Source: CAD feature listing. Evaluate the final solid. Frame: model axes, mm. A direction names the side the tool comes from. Coordinates: 2 decimals unless noted, no trailing zeros. Order: outer loops, then holes, each group sorted by start corner. A loop starts at its lowest first (then second) coordinate and runs counter-clockwise, first axis right, second up.
```python
from build123d import *

# Parameters (mm, degrees)
F1_DEPTH  = 50.8
F2_R      = 3.9624
F3_SIZE   = 6.35
F5_DEPTH  = 44.451
F7_D      = 13.0302
F9_DEPTH  = 69.851
F10_R     = 29.21
F11_DEPTH = 29.591
F12_SIZE  = 4.19099
F14_DEPTH = 14.9870001
F16_DEPTH = 16.764
F17_R     = 6.35
F18_DEPTH = 69.851


# Not quite as in the source:
# - a fillet or chamfer is up to 0.001 mm smaller than in the source, because OpenCascade refuses the exact size


with BuildPart() as f1:
    # F0 (on Top) → F1 (new body)
    with BuildSketch(Plane.XY):
        Polygon((44.45, 120.65), (0, 120.65), (0, 0), (0, -21.59), (0, -73.9648), (14.986, -73.9648), (14.986, 26.2809675187), (31.75, 26.2809675187), (31.75, -21.59), (69.85, -21.59), (69.85, 0), (44.45, 0), align=None)
    extrude(amount=F1_DEPTH)

    # F2
    f2_edges = [f1.edges().sort_by_distance(p)[0] for p in [
        (44.45, 0, 25.4),
        (14.986, 26.280968, 25.4),
        (31.75, 26.280968, 25.4),
    ]]
    fillet(f2_edges, radius=F2_R)

    # F3
    f3_edges = [f1.edges().sort_by_distance(p)[0] for p in [
        (22.225, 120.65, 50.8),
        (22.225, 120.65, 0),
    ]]
    chamfer(f3_edges, length=F3_SIZE)

    # F4 (on face) → F5 (cut, through all)
    with BuildSketch(Plane.YZ.offset(44.45)):
        with BuildLine():
            Line((120.65, 38.0365), (107.8865, 38.0365))
            ThreePointArc((107.8865, 38.0365), (95.25, 25.4), (107.8865, 12.7635))
            Line((107.8865, 12.7635), (120.65, 12.7635))
            Line((120.65, 12.7635), (120.65, 38.0365))
        make_face()
    extrude(amount=-F5_DEPTH, mode=Mode.SUBTRACT)

    # F7 (through all)
    with Locations(Plane.YZ.offset(69.85)):
        with Locations((7.62, 12.954)):
            Hole(F7_D / 2)

    # F8 (on face) → F9 (cut, through all)
    with BuildSketch(Plane(origin=(0, 0, 0), x_dir=(0, -1, 0), z_dir=(-1, 0, 0))):
        with BuildLine():
            Line((-8.8916366414, 50.8), (-70.4833633586, 50.8))
            Line((-70.4833633586, 50.8), (-61.6845452561, 35.56))
            ThreePointArc((-61.6845452561, 35.56), (-39.6875, 22.86), (-17.6904547439, 35.56))
            Line((-17.6904547439, 35.56), (-8.8916366414, 50.8))
        make_face()
    extrude(amount=-F9_DEPTH, mode=Mode.SUBTRACT)

    # F10 (on face) → F11 (cut)
    with BuildSketch(Plane.YZ.offset(69.85)):
        with Locations((39.6875, 48.26)):
            Circle(F10_R)
    extrude(amount=-F11_DEPTH, mode=Mode.SUBTRACT)

    # F12 (size 4.191 in the source; OpenCascade refuses exactly that, so slightly less here)
    f12_edges = [f1.edges().sort_by_distance(p)[0] for p in [
        (44.45, 39.6875, 19.05),
    ]]
    chamfer(f12_edges, length=F12_SIZE)

    # F13 (on face) → F14 (cut, through all)
    with BuildSketch(Plane.YZ.offset(14.986)):
        with BuildLine():
            Line((-73.9648, 50.8), (-73.9648, 0))
            ThreePointArc((-73.9648, 0), (-67.8661098873, 9.9669221787), (-65.0748, 21.3133818873))
            Line((-65.0748, 21.3133818873), (-62.4950551894, 50.8))
            Line((-62.4950551894, 50.8), (-73.9648, 50.8))
        make_face()
    extrude(amount=-F14_DEPTH, mode=Mode.SUBTRACT)

    # F15 (on face) → F16 (cut, through all)
    with BuildSketch(Plane.YZ.offset(14.986)):
        Polygon((11.9264439221, 19.6698105436), (22.8565887415, 19.6698105436), (41.9241071546, 38.7373289567), (11.9264439221, 38.7373289567), align=None)
    extrude(amount=F16_DEPTH, mode=Mode.SUBTRACT)

    # F17 (on face) → F18 (cut, through all)
    with BuildSketch(Plane(origin=(0, 0, 0), x_dir=(0, -1, 0), z_dir=(-1, 0, 0))):
        with Locations((33.655, 12.7)):
            Circle(F17_R)
        with Locations((33.655, 41.275)):
            Circle(F17_R)
    extrude(amount=-F18_DEPTH, mode=Mode.SUBTRACT)


solid = f1.part
```
Q1. Section query A-A on x = 5. Give the number of separate pieces and of enclosed holes in the cut face, plus the area to 3 significant figures.
Solutions:
separate pieces: 1
enclosed holes: 3
area: 7,260 mm2
Q2. Pull-direction query (Y, two-part tool) for faces 1 (the cylindrical face through (19.848, 40.06, 22.863)), 2 (the flat face through (40.259, 40, 22)), 3 (the flat face through (23.251, 26.962, 23.775)), 4 (the flat face through (0, 25, 25)); classes: pulls with the +Y half, pulls with the -Y half, needs draft (parallel to the pull), parting line crosses it, or undercut.
Solutions:
face 1: undercut
face 2: undercut
face 3: pulls with the -Y half
face 4: needs draft
Q3. Pin query (flat end, axial travel): P1, Ø4, axis at x = 18, y = -49.5, coming from the -Z side; P2, Ø12, axis at y = 47, z = 16, coming from the +X side; P3, Ø7, axis at x = 23, z = 10, coming from the -Y side; P4, Ø23, axis at y = 35, z = 31.5, coming from the +X side. Return the tip coordinate at first contact, or that it passes through.
Solutions:
P1: passes through
P2: stops at x = 44.45
P3: stops at y = 26.28
P4: stops at x = 40.26
Q4. Section query B-B on z = 4. Output: boundary loops of the cut face in (x, y).
Solutions:
outline: (0, -71) - (14.99, -71) - (14.99, 22.32) arc R3.96 cw to (18.95, 26.28) - (27.79, 26.28) arc R3.96 cw to (31.75, 22.32) - (31.75, -21.59) - (69.85, -21.59) - (69.85, 0) - (48.41, 0) arc R3.96 cw to (44.45, 3.96) - (44.45, 118.3) - (0, 118.3) - close
Q5. Set-up query: faces 5 (the flat face through (23, 26.281, 11)), 6 (the flat face through (22, 93, 50.8)), 7 (the flat face through (44.45, 74, 19)). Return all of +Z, -Z, +X, -X, +Y, -Y with unobstructed straight access to the full face (end or side cutting, diameter ignored); none if empty.
Solutions:
face 5: +Z, -Z, -Y
face 6: +Z, +X, -X, +Y, -Y
face 7: +Z, -Z, +X, +Y
Q6. Section query D-D on x = 35. Output: boundary loops of the cut face in (y, z).
Solutions:
outline: (-21.59, 0) - (114.3, 0) - (120.65, 6.35) - (120.65, 12.76) - (107.89, 12.76) arc R12.64 cw to (107.89, 38.04) - (120.65, 38.04) - (120.65, 44.45) - (114.3, 50.8) - (70.48, 50.8) - (61.68, 35.56) arc R25.4 cw to (17.69, 35.56) - (8.89, 50.8) - (-21.59, 50.8) - close; hole circle Ø13.03 at (7.62, 12.95)
Q7. Material intervals for line 1 along X through (y, z) = (-11.5, 35.5); line 2 along Z through (x, y) = (37, 7); line 3 along Y through (x, z) = (12, 9.5), sorted ascending.
Solutions:
line 1: x = 0 to 14.99, 31.75 to 69.85
line 2: z = 0 to 6.47, 19.44 to 50.8
line 3: y = -68.06 to -39.14, -28.17 to 2.1, 13.14 to 120.65
Q8. Section query C-C on x = 17. Output: boundary loops of the cut face in (y, z), plus the area to 3 significant figures.
Solutions:
outline: (25.77, 0) - (114.3, 0) - (120.65, 6.35) - (120.65, 12.76) - (107.89, 12.76) arc R12.64 cw to (107.89, 38.04) - (120.65, 38.04) - (120.65, 44.45) - (114.3, 50.8) - (70.48, 50.8) - (61.68, 35.56) arc R25.4 cw to (28.6, 25.41) - (25.77, 22.58) - close
area: 3,230 mm2
